Design review of the part built by this model. Coordinates are the model's own, in mm. Face numbers are marked on the shaded views. A direction names the side the tool comes from. Round coordinates to 2 decimals unless told otherwise and drop trailing zeros. Write each loop counter-clockwise with the first axis right and the second up, starting at its lowest first coordinate (ties: lowest second). Pieces come first, ordered by that corner, then holes. Notation, with made-up numbers: M 23.25,-9.75 L 50.25,-9.75 A35 cw 50.25,23.25 Z; hole C 70,46 d10. An arc over 180 degrees is marked long. One line per question, with ' | ' between items. Start each with the question number.
Item 1: Insertion check: pin 1 Ø1.9 at (y, z) = (8, 4.5) entering from -X; pin 2 Ø1.5 at (x, y) = (-0.5, 3.5) entering from -Z; pin 3 Ø5 at (y, z) = (4.5, 1.5) entering from -X. Each pin has a flat end and moves straight along its axis. Give the tip position at first contact, or say it passes through.
Item 2: For L1, parallel to Z at x = 0, y = 9.25; L2, parallel to Y at x = 0, z = 4.25; L3, parallel to X at y = 4.5, z = 4.25, list the stretches that pass through material, from the lowest coordinate up.
Item 3: Machinability: for the marked faces 4, 5, 6, 7 and 8, which of the approach directions +Z, -Z, +X, -X, +Y, -Y give a long, thin tool a straight path to every point of the face, cutting with its end or side? Answer none if there is none.
Item 4: Add section A-A, the plane x = 0. State the section outline as (y, z) points, and give its area (3 significant figures).
Item 5: Draft analysis for pull direction X (two halves, no side actions). For the marked faces 1, 2 and 3, state which applies: released by +X, released by -X, zero draft, split by the parting line, or undercut.
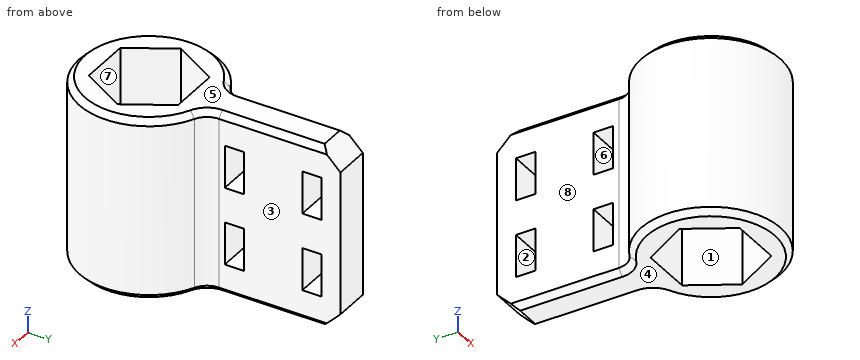
```python
from build123d import *

# Parameters (mm, degrees)
SKETCH2_R           = 3.6
SKETCH2_R_2         = 1.625
BOSS_EXTRUDE1_DEPTH = 9.4
BOSS_EXTRUDE2_DEPTH = 9.4
SKETCH4_W           = 2.2
SKETCH4_H           = 1
CUT_EXTRUDE2_DEPTH  = 10
CHAMFER2_SIZE       = 1
FILLET1_R           = 1
CUT_EXTRUDE3_DEPTH  = 10
CHAMFER1_SIZE       = 0.3


with BuildPart() as part:
    # Sketch2 → Boss-Extrude1 (new body)
    with BuildSketch(Plane.XY):
        Circle(SKETCH2_R)
        Circle(SKETCH2_R_2, mode=Mode.SUBTRACT)
    extrude(amount=BOSS_EXTRUDE1_DEPTH)

    # Sketch3 → Boss-Extrude2 (add)
    with BuildSketch(Plane.XY.offset(9.4)):
        with BuildLine():
            Line((-0.9375, 10.44191444), (-0.9375, 3.475786781))
            ThreePointArc((-0.9375, 3.475786781), (0, 3.6), (0.9375, 3.475786781))
            Line((0.9375, 3.475786781), (0.9375, 10.44191444))
            Line((0.9375, 10.44191444), (-0.9375, 10.44191444))
        make_face()
    extrude(amount=-BOSS_EXTRUDE2_DEPTH)

    # Sketch4 → Cut-Extrude2 (cut)
    with BuildSketch(Plane.ZY.offset(0.9375)):
        with Locations((2.7, 8.975786781)):
            Rectangle(SKETCH4_W, SKETCH4_H)
        with Locations((6.7, 8.975786781)):
            Rectangle(SKETCH4_W, SKETCH4_H)
        with Locations((2.7, 4.975786781)):
            Rectangle(SKETCH4_W, SKETCH4_H)
        with Locations((6.7, 4.975786781)):
            Rectangle(SKETCH4_W, SKETCH4_H)
    extrude(amount=-CUT_EXTRUDE2_DEPTH, mode=Mode.SUBTRACT)

    # Chamfer2
    chamfer2_edges = [part.edges().sort_by_distance(p)[0] for p in [
        (0, 10.44191444, 0),
        (0, 10.44191444, 9.4),
    ]]
    chamfer(chamfer2_edges, length=CHAMFER2_SIZE)

    # Fillet1
    fillet1_edges = [part.edges().sort_by_distance(p)[0] for p in [
        (0.9375, 3.475786781, 4.7),
        (-0.9375, 3.475786781, 4.7),
    ]]
    fillet(fillet1_edges, radius=FILLET1_R)

    # Sketch5 → Cut-Extrude3 (cut)
    with BuildSketch(Plane(origin=(0, 0, 0), x_dir=(-1, 0, 0), z_dir=(0, 0, -1))):
        Polygon((1.327905619, 2.3), (-1.327905619, 2.3), (-2.655811238, 0), (-1.327905619, -2.3), (1.327905619, -2.3), (2.655811238, 0), align=None)
    extrude(amount=-CUT_EXTRUDE3_DEPTH, mode=Mode.SUBTRACT)

    # Chamfer1
    chamfer1_edges = [part.edges().sort_by_distance(p)[0] for p in [
        (0.9375, 6.806987766, 0),
        (-0.9375, 6.806987766, 0),
        (0, -3.6, 0),
        (0, -3.6, 9.4),
        (0.9375, 6.806987766, 9.4),
        (-0.9375, 6.806987766, 9.4),
        (1.094530353, 3.634099965, 9.4),
        (1.094530353, 3.634099965, 0),
        (-1.094530353, 3.634099965, 9.4),
        (-1.094530353, 3.634099965, 0),
    ]]
    chamfer(chamfer1_edges, length=CHAMFER1_SIZE)


solid = part.part
```
Computed values:
1) pin 1: stops at x = -0.94 | pin 2: stops at z = 0 | pin 3: stops at x = -2.99
2) L1: z = 0 to 1.6, 3.8 to 5.6, 7.8 to 9.4 | L2: y = -3.6 to -2.3, 2.3 to 10.44 | L3: x = -0.94 to 0.94
3) face 4: -Z, +X, -X, +Y, -Y | face 5: +Z, +X, -X, +Y, -Y | face 6: +X, -X | face 7: +Z, -Z | face 8: +Z, -Z, -X, +Y
4) outline: M -3.6,0.3 L -3.3,0 L -2.3,0 L -2.3,9.4 L -3.3,9.4 L -3.6,9.1 Z; M 2.3,0 L 9.44,0 L 10.44,1 L 10.44,8.4 L 9.44,9.4 L 2.3,9.4 Z; hole M 4.48,1.6 L 5.48,1.6 L 5.48,3.8 L 4.48,3.8 Z; hole M 4.48,5.6 L 5.48,5.6 L 5.48,7.8 L 4.48,7.8 Z; hole M 8.48,1.6 L 9.48,1.6 L 9.48,3.8 L 8.48,3.8 Z; hole M 8.48,5.6 L 9.48,5.6 L 9.48,7.8 L 8.48,7.8 Z | area: 78.9 mm^2
5) face 1: undercut | face 2: zero draft | face 3: released by +X
